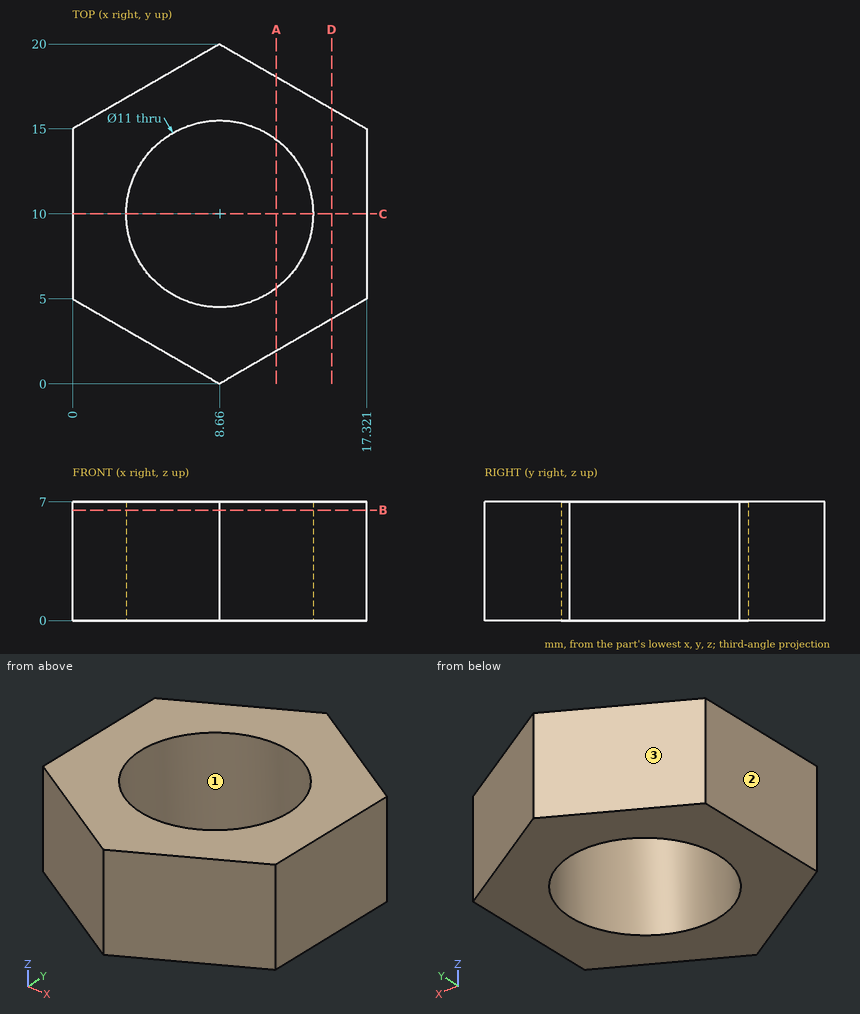
Study the drawing (mm; zero at the part's minimum x, y, z) and answer. Coordinates: 2 decimals unless noted, no trailing zeros. Order: outer loops, then holes, each group sorted by start corner. A loop starts at its lowest first (then second) coordinate and runs counter-clockwise, first axis right, second up. Notation, with made-up numbers: M 16,66 L 45,66 A8 cw 45,77 Z; hole C 75,-23 d2. An arc over 180 degrees is marked long. Answer as a JSON object with one key per item and string values. Group by question number.
1. Section C-C on y = 10 is taken. Write down the section's boundary in (x, z).
2. Straight lines are drawn through the part: line 1 (X direction, y = 10, z = 3.75); line 2 (Y direction, x = 10, z = 5) (1 decimal); line 3 (Y direction, x = 12.75, z = 2.25) (1 decimal). For each, find the intervals that lie inside material, in ascending order.
3. Section B-B on z = 6.5 is taken. Write down the section's boundary in (x, y), then the cut area to 3 significant figures.
4. Section A-A on x = 12 is taken. Write down the section's boundary in (y, z).
5. Determine the mould class of the marked faces 1, 2 and 3 for opening direction Y: released by +Y, released by -Y, zero draft, split by the parting line, or undercut.
6. Section D-D on x = 15.25 is taken. Write down the section's boundary in (y, z) (1 decimal).
Values follow:
{
 "1": {"outline": "M 0,0 L 3.16,0 L 3.16,7 L 0,7 Z; M 14.16,0 L 17.32,0 L 17.32,7 L 14.16,7 Z"},
 "2": {"line 1": "0 to 3.16, 14.16 to 17.32", "line 2": "0.8 to 4.7, 15.3 to 19.2", "line 3": "2.4 to 6.3, 13.7 to 17.6"},
 "3": {"outline": "M 0,5 L 8.66,0 L 17.32,5 L 17.32,15 L 8.66,20 L 0,15 Z; hole C 8.66,10 d11", "area": "165 mm2"},
 "4": {"outline": "M 1.93,0 L 5.63,0 L 5.63,7 L 1.93,7 Z; M 14.37,0 L 18.07,0 L 18.07,7 L 14.37,7 Z"},
 "5": {"face 1": "undercut", "face 2": "zero draft", "face 3": "released by +Y"},
 "6": {"outline": "M 3.8,0 L 16.2,0 L 16.2,7 L 3.8,7 Z"}
}
